```python
from build123d import *

# Parameters (mm, degrees)
SKETCH1_R                = 17.145
SKETCH1_R_2              = 3.937
SKETCH1_R_3              = 1.524
BOSS_EXTRUDE1_DEPTH      = 2.54
SKETCH2_R                = 3.937
BOSS_EXTRUDE2_DEPTH      = 73.66
BOSS_EXTRUDE2_DEPTH_BACK = 2.54
BOSS_EXTRUDE8_DEPTH      = 3.81
BOSS_EXTRUDE8_DEPTH_BACK = 52.07
SKETCH10_R               = 3.81
BOSS_EXTRUDE9_DEPTH      = 19.05
CUT_EXTRUDE1_DEPTH       = 46.99
FILLET3_R                = 2.54


with BuildPart() as part:
    # Sketch1 → Boss-Extrude1 (new body)
    with BuildSketch(Plane.XY):
        Circle(SKETCH1_R)
        Circle(SKETCH1_R_2, mode=Mode.SUBTRACT)
        with Locations((0, 7.874)):
            Circle(SKETCH1_R_3, mode=Mode.SUBTRACT)
        with Locations((0, -7.874)):
            Circle(SKETCH1_R_3, mode=Mode.SUBTRACT)
        with Locations((-9.398, 0)):
            Circle(SKETCH1_R_3, mode=Mode.SUBTRACT)
        with Locations((9.398, 0)):
            Circle(SKETCH1_R_3, mode=Mode.SUBTRACT)
    extrude(amount=BOSS_EXTRUDE1_DEPTH)

    # Sketch2 → Boss-Extrude2 (add, two sides)
    with BuildSketch(Plane.XY.offset(2.54)) as boss_extrude2_sk:
        Circle(SKETCH2_R)
    extrude(amount=BOSS_EXTRUDE2_DEPTH)
    extrude(boss_extrude2_sk.sketch, amount=-BOSS_EXTRUDE2_DEPTH_BACK)

    # Sketch9 → Boss-Extrude8 (add, two sides)
    with BuildSketch(Plane.XY.offset(76.2)) as boss_extrude8_sk:
        with BuildLine():
            Line((17.310299419, 6.04983425), (-8.943054295, -16.008395932))
            ThreePointArc((-8.943054295, -16.008395932), (-18.105957698, -15.212737654), (-17.310299419, -6.04983425))
            Line((-17.310299419, -6.04983425), (8.943054295, 16.008395932))
            ThreePointArc((8.943054295, 16.008395932), (18.105957698, 15.212737654), (17.310299419, 6.04983425))
        make_face()
    extrude(amount=BOSS_EXTRUDE8_DEPTH)
    extrude(boss_extrude8_sk.sketch, amount=-BOSS_EXTRUDE8_DEPTH_BACK)

    # Sketch10 → Boss-Extrude9 (add)
    with BuildSketch(Plane.XY.offset(80.01)):
        with Locations((13.126676857, 11.029115091)):
            Circle(SKETCH10_R)
        with Locations((-13.126676857, -11.029115091)):
            Circle(SKETCH10_R)
    extrude(amount=BOSS_EXTRUDE9_DEPTH)

    # Sketch11 → Cut-Extrude1 (cut)
    with BuildSketch(Plane.XY.offset(80.01)):
        Polygon((3.374041748, 12.335861743), (-12.725218051, -1.275330633), (-3.374041748, -12.335861743), (12.725218051, 1.275330633), align=None)
    extrude(amount=-CUT_EXTRUDE1_DEPTH, mode=Mode.SUBTRACT)

    # Fillet3
    fillet3_edges = [part.edges().sort_by_distance(p)[0] for p in [
        (-3.937, 0, 24.13),
    ]]
    fillet(fillet3_edges, radius=FILLET3_R)


solid = part.part
```
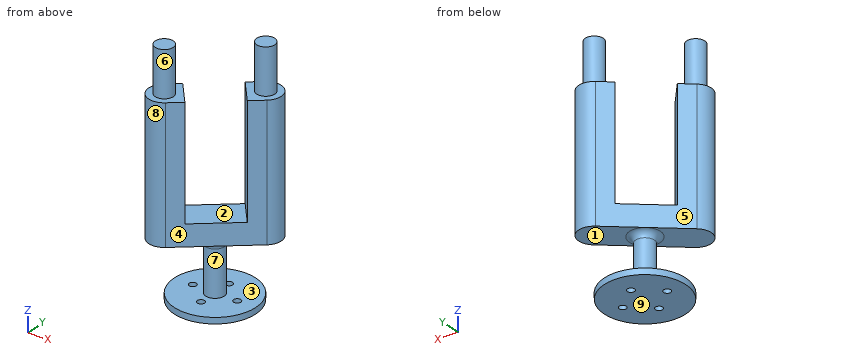
Geometry check sheet. Reference: the model listing, model coordinates, mm. Face numbers are marked on the shaded views. A direction names the side the tool comes from. Coordinates: 2 decimals unless noted, no trailing zeros. Write each loop counter-clockwise with the first axis right and the second up, starting at its lowest first coordinate (ties: lowest second). Pieces come first, ordered by that corner, then holes. Notation, with made-up numbers: M 70.5,82 L 85.5,82 A20 ccw 85.5,103 Z; hole C -33.75,15 d8. An arc over 180 degrees is marked long. One line per item, written item: value. Start each with the question number.
(1) Depth check by flat-ended pin: pin 1 (1.8 mm diameter, centred on x = 0, y = 7.874, fed in from -Z); pin 2 (11.5 mm diameter, centred on x = -2.5, y = -1, fed in from +Z); pin 3 (12 mm diameter, centred on x = -3, y = -7, fed in from +Z). Enter the tip coordinate at first touch or a pass-through.
(2) Sectioned sample at A-A, the plane z = 45.5. Enter the section's corners in (x, y), and give its area (3 significant figures).
(3) Sectioned sample at C-C, the plane x = 0. Enter the section's corners in (y, z) (3 decimals), and give its area (3 significant figures).
(4) Tool access check on the marked faces 5, 6, 7, 8 and 9. Record the directions out of +Z, -Z, +X, -X, +Y, -Y that give a thin tool (end or side, any length) a straight path to the whole face; none if there is none.
(5) Sectioned sample at B-B, the plane y = 13. Enter the section's corners in (x, z).
(6) Scan lines: line 1 along Y through (x, z) = (0, 1.6) (3 decimals); line 2 along Z through (x, y) = (15.5, 5.5); line 3 along Z through (x, y) = (3.5, -10). Record each from-to range of solid material in increasing order. Write a range as [from, to].
(7) Sectioned sample at D-D, the plane y = 0. Enter the section's corners in (x, z) (3 decimals).
(8) Release check for a two-part mould opening along Z. For the marked faces 1, 2, 3 and 4 record: released by +Z, released by -Z, zero draft, split by the parting line, or undercut.
Filled sheet:
1. pin 1: z = 24.13
1. pin 2: z = 33.02
1. pin 3: z = 80.01
2. outline: M -17.31,-6.05 A6.5 ccw -8.94,-16.01 L -3.87,-11.75 L -12.27,-1.81 Z; M 3.87,11.75 L 12.27,1.81 L 17.31,6.05 A6.5 ccw 8.94,16.01 Z
2. area: 305 mm²
3. outline: M -17.145,0 L -9.398,0 L -9.398,2.54 L -17.145,2.54 Z; M -8.494,24.13 L -6.477,24.13 A2.54 cw -3.937,21.59 L -3.937,2.54 L -6.35,2.54 L -6.35,0 L 6.35,0 L 6.35,2.54 L 3.937,2.54 L 3.937,21.59 A2.54 cw 6.477,24.13 L 8.494,24.13 L 8.494,33.02 L -8.494,33.02 Z; M 9.398,0 L 17.145,0 L 17.145,2.54 L 9.398,2.54 Z
3. area: 395 mm²
4. face 5: +Z, -X, +Y
4. face 6: +Z
4. face 7: none
4. face 8: +Z, -Z
4. face 9: -Z, +X, -X, +Y, -Y
5. outline: M -11.18,0 L 11.18,0 L 11.18,2.54 L -11.18,2.54 Z; M 5.36,24.13 L 19.32,24.13 L 19.32,80.01 L 16.39,80.01 L 16.39,99.06 L 9.87,99.06 L 9.87,80.01 L 5.36,80.01 Z
6. line 1: [-17.145, -9.398], [-6.35, 6.35], [9.398, 17.145]
6. line 2: [0, 2.54], [24.13, 80.01]
6. line 3: [0, 2.54]
7. outline: M -17.145,0 L -10.922,0 L -10.922,2.54 L -17.145,2.54 Z; M -10.11,24.13 L -6.477,24.13 A2.54 cw -3.937,21.59 L -3.937,2.54 L -7.874,2.54 L -7.874,0 L 7.874,0 L 7.874,2.54 L 3.937,2.54 L 3.937,21.59 A2.54 cw 6.477,24.13 L 10.11,24.13 L 10.11,33.02 L -10.11,33.02 Z; M 10.922,0 L 17.145,0 L 17.145,2.54 L 10.922,2.54 Z
8. face 1: undercut
8. face 2: released by +Z
8. face 3: undercut
8. face 4: zero draft
